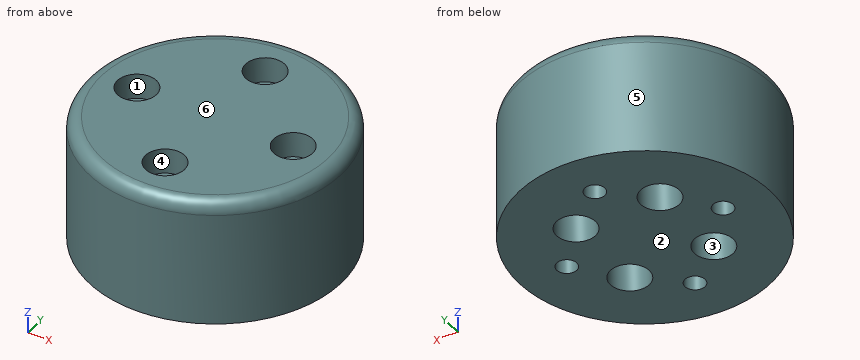
```python
from build123d import *

# Parameters (mm, degrees)
SKETCH_1_R          = 20
SKETCH_1_R_2        = 1.6
EXTRUDE_1_DEPTH     = 20
SKETCH_2_R          = 3.1
CUT_EXTRUDE_1_DEPTH = 4
SKETCH_3_R          = 3.1
CUT_EXTRUDE_2_DEPTH = 5
FILLET_1_R          = 2


with BuildPart() as part:
    # 草图1 → 凸台-拉伸1 (new body)
    with BuildSketch(Plane.XY):
        Circle(SKETCH_1_R)
        with Locations((12.5, 0)):
            Circle(SKETCH_1_R_2, mode=Mode.SUBTRACT)
        with Locations((0, -12.5)):
            Circle(SKETCH_1_R_2, mode=Mode.SUBTRACT)
        with Locations(Location((-12.5, 0, 0), (0, 0, 180))):
            Circle(SKETCH_1_R_2, mode=Mode.SUBTRACT)
        with Locations(Location((0, 12.5, 0), (0, 0, 180))):
            Circle(SKETCH_1_R_2, mode=Mode.SUBTRACT)
    extrude(amount=EXTRUDE_1_DEPTH)

    # 草图2 → 切除-拉伸1 (cut)
    with BuildSketch(Plane.XY.offset(20)):
        with Locations((-12.5, 0)):
            Circle(SKETCH_2_R)
        with Locations((0, -12.5)):
            Circle(SKETCH_2_R)
        with Locations((12.5, 0)):
            Circle(SKETCH_2_R)
        with Locations((0, 12.5)):
            Circle(SKETCH_2_R)
    extrude(amount=-CUT_EXTRUDE_1_DEPTH, mode=Mode.SUBTRACT)

    # 草图3 → 切除-拉伸2 (cut)
    with BuildSketch(Plane(origin=(0, 0, 0), x_dir=(-1, 0, 0), z_dir=(0, 0, -1))):
        with Locations((-6.717514421, 6.717514421)):
            Circle(SKETCH_3_R)
        with Locations((6.717514421, 6.717514421)):
            Circle(SKETCH_3_R)
        with Locations((6.717514421, -6.717514421)):
            Circle(SKETCH_3_R)
        with Locations((-6.717514421, -6.717514421)):
            Circle(SKETCH_3_R)
    extrude(amount=-CUT_EXTRUDE_2_DEPTH, mode=Mode.SUBTRACT)

    # 圆角1
    fillet_1_edges = [part.edges().sort_by_distance(p)[0] for p in [
        (-20, 0, 20),
    ]]
    fillet(fillet_1_edges, radius=FILLET_1_R)


solid = part.part
```
The listing builds one solid part. Answer for the finished solid, in the listing's coordinates (mm). Face numbers are marked on the shaded views. A direction names the side the tool comes from. Give positions to 0.01 mm unless a question says otherwise; leave off trailing zeros. Write each loop counter-clockwise with the first axis right and the second up, starting at its lowest first coordinate (ties: lowest second). Pieces come first, ordered by that corner, then holes. Notation, with made-up numbers: (25.5, 66) - (68.5, 66) arc R20 ccw to (68.5, 104) - close; hole circle Ø5 at (-19.5, -6.5). An arc over 180 degrees is marked (long way). Use one line per item in the form item = value. Start each with the question number.
1) Find section A-A on x = 0. Determine the outline of the cut face in (y, z).
2) A tool of negligible diameter and unlimited length cuts with its end or side. For the marked faces 1, 2 and 3, from which of +Z, -Z, +X, -X, +Y, -Y can it reach the whole face along a straight path? Write none if from no direction.
3) The mould has two halves that part along Y. Classify the marked faces 4, 5 and 6: pulls with the +Y half, pulls with the -Y half, needs draft (parallel to the pull), parting line crosses it, or undercut.
4) Flat-ended cylindrical pins translate along their axes: pin 1 Ø3 at (x, y) = (6, 8) entering from -Z; pin 2 Ø5 at (y, z) = (-7.5, 16.5) entering from +X; pin 3 Ø5 at (x, y) = (-6, 7) entering from -Z; pin 4 Ø1 at (x, z) = (6, 7) entering from -Y. Find the tip coordinate at first contact, or state that the pin passes through.
5) Consider line 1 along Y through (x, z) = (0, 5.25); line 2 along X through (y, z) = (-12.5, 8.25); line 3 along Y through (x, z) = (6, 3). Determine where each line is inside the solid, lowest interval first. Write a range as from..to.
6) Find section C-C on z = 10.5. Determine the outline of the cut face in (x, y), plus the area to 3 significant figures.
Geometry results:
q1.outline = (-20, 0) - (-14.1, 0) - (-14.1, 16) - (-15.6, 16) - (-15.6, 20) - (-18, 20) arc R2 ccw to (-20, 18) - close; (-10.9, 0) - (10.9, 0) - (10.9, 16) - (9.4, 16) - (9.4, 20) - (-9.4, 20) - (-9.4, 16) - (-10.9, 16) - close; (14.1, 0) - (20, 0) - (20, 18) arc R2 ccw to (18, 20) - (15.6, 20) - (15.6, 16) - (14.1, 16) - close
q2.face_1 = +Z
q2.face_2 = -Z, +X, -X, +Y, -Y
q2.face_3 = -Z
q3.face_4 = undercut
q3.face_5 = parting line crosses it
q3.face_6 = needs draft
q4.pin_1 = 5
q4.pin_2 = 19.36
q4.pin_3 = 0
q4.pin_4 = -19.23
q5.line_1 = -20..-14.1, -10.9..10.9, 14.1..20
q5.line_2 = -15.61..-1.6, 1.6..15.61
q5.line_3 = -19.08..-9.73, -3.7..3.7, 9.73..19.08
q6.outline = circle Ø40 at (0, 0); hole circle Ø3.2 at (-12.5, 0); hole circle Ø3.2 at (0, -12.5); hole circle Ø3.2 at (0, 12.5); hole circle Ø3.2 at (12.5, 0)
q6.area = 1,220 mm2
